Geometry check sheet. Reference: the model listing, model coordinates, mm. A direction names the side the tool comes from. Coordinates: 2 decimals unless noted, no trailing zeros. Write each loop counter-clockwise with the first axis right and the second up, starting at its lowest first coordinate (ties: lowest second). Pieces come first, ordered by that corner, then holes. Notation, with made-up numbers: (0, 74) -> (53, 74) arc R26 ccw to (53, 107) -> close; hole circle Ø1 at (6, -28.5). An arc over 180 degrees is marked (long way). One line per question, with ' | ' between items.
from build123d import *

# Parameters (mm, degrees)
EXTRUDE_1_DEPTH     = 5
SKETCH_2_R          = 8.75
EXTRUDE_2_DEPTH     = 30
SKETCH_4_R          = 4.5
CUT_EXTRUDE_1_DEPTH = 25
SKETCH_5_R          = 4
EXTRUDE_3_DEPTH     = 15


with BuildPart() as part:
    # 草图1 → 凸台-拉伸1 (new body)
    with BuildSketch(Plane(origin=(0, 0, 0), x_dir=(1, 0, 0), z_dir=(0, 1, 0))):
        Polygon((0, 4.618802154), (-4, 2.309401077), (-4, -2.309401077), (0, -4.618802154), (4, -2.309401077), (4, 2.309401077), align=None)
    extrude(amount=EXTRUDE_1_DEPTH)

    # 草图2 → 凸台-拉伸2 (add)
    with BuildSketch(Plane(origin=(0, 5, 0), x_dir=(1, 0, 0), z_dir=(0, 1, 0))):
        with Locations(Location((0, 0, 0), (0, 0, 270))):
            Circle(SKETCH_2_R)
    extrude(amount=EXTRUDE_2_DEPTH)

    # 草图3 → 旋转1 (revolve)
    with BuildSketch(Plane.XY):
        with BuildLine():
            ThreePointArc((0, 31), (11, 42), (0, 53))
            Line((0, 53), (0, 31))
        make_face()
    revolve(axis=Axis((0, 53, 0), (0, -1, 0)))

    # 草图4 → 切除-拉伸1 (cut, symmetric)
    with BuildSketch(Plane.XY):
        with Locations((0, 42)):
            Circle(SKETCH_4_R)
    extrude(amount=CUT_EXTRUDE_1_DEPTH, both=True, mode=Mode.SUBTRACT)

    # 草图5 → 凸台-拉伸3 (add)
    with BuildSketch(Plane.XZ):
        with Locations(Location((0, 0, 0), (0, 0, 120))):
            Circle(SKETCH_5_R)
    extrude(amount=EXTRUDE_3_DEPTH)


solid = part.part
1. Cross-section at D-D on z = -6. Record the boundary of the cut face in (x, y).
Worked answers:
outline: (-6.37, 5) -> (6.37, 5) -> (6.37, 35) -> (6, 35) arc R9.22 ccw (long way) to (-6, 35) -> (-6.37, 35) -> close; hole circle Ø9 at (0, 42)
2. Cross-section at C-C on y = 8. Record the boundary of the cut face in (x, z).
Worked answers:
outline: circle Ø17.5 at (0, 0)
3. Go/stop test with flat-tipped pins: P1, Ø1, axis at x = 7.5, y = 9.5, coming from the -Z side; P2, Ø1, axis at y = 17, z = -4, coming from the +X side; P3, Ø2, axis at x = 6, z = 6.5, coming from the +Y side; P4, Ø9, axis at x = 3.5, z = -4.5, coming from the -Y side. Record where each tip stops, or that it passes through.
Worked answers:
P1: z = -5.25 | P2: x = 8.02 | P3: y = 49.71 | P4: y = -15
4. Material ranges on line 1 (Y direction, x = 0, z = -0.5); line 2 (Y direction, x = -2.25, z = 8); line 3 (Z direction, x = 0, y = -4.5), recorded low to high. Write a range as from..to.
Worked answers:
line 1: -15..37.5, 46.5..52.99 | line 2: 5..38.1, 45.9..49.21 | line 3: -4..4
5. Tool access check on faces 1 (the face through (3.6, 0, 2.1)), 2 (the face through (3.695, -7.395, -1.532)), 3 (the face through (-2.028, 2.465, 3.448)), 4 (the face through (4, 2, 0)), 5 (the face through (2.028, 2.465, -3.448)). Record the directions out of +Z, -Z, +X, -X, +Y, -Y that give a thin tool (end or side, any length) a straight path to the whole face; none if there is none.
Worked answers:
face 1: +Z, +X, -Y | face 2: -Y | face 3: +Z, -X, -Y | face 4: +Z, -Z, +X, -Y | face 5: -Z, +X, -Y
6. Cross-section at B-B on y = 42. Record the boundary of the cut face in (x, z), and give its area (3 significant figures).
Worked answers:
outline: (-4.5, -10.04) -> (-4.5, 10.04) arc R11 ccw to start; (4.5, -10.04) arc R11 ccw to (4.5, 10.04) -> close | area: 188 mm²
7. Cross-section at A-A on z = 6.75. Record the boundary of the cut face in (x, y).
Worked answers:
outline: (-5.57, 5) -> (5.57, 5) -> (5.57, 35) -> (5.14, 35) arc R8.69 ccw (long way) to (-5.14, 35) -> (-5.57, 35) -> close; hole circle Ø9 at (0, 42)
